```python
from build123d import *

# Parameters (mm, degrees)
BOSS_EXTRUDE1_DEPTH = 6.35
SKETCH3_R           = 3.302
SKETCH3_R_2         = 3.175
SKETCH3_R_3         = 7.14375
SKETCH3_R_4         = 1.905
CUT_EXTRUDE1_DEPTH  = 7.62
SKETCH5_R           = 2.667
SKETCH5_R_2         = 3.175
CUT_EXTRUDE2_DEPTH  = 7.62


with BuildPart() as part:
    # Sketch1 → Boss-Extrude1 (new body)
    with BuildSketch(Plane(origin=(0, 0, 0), x_dir=(1, 0, 0), z_dir=(0, 1, 0))):
        Polygon((0, 0), (495.3, 0), (495.3, -48.8188), (647.7, -48.8188), (647.7, 154.3812), (-152.4, 154.3812), (-152.4, -48.8188), (0, -48.8188), align=None)
    extrude(amount=BOSS_EXTRUDE1_DEPTH)

    # Sketch3 → Cut-Extrude1 (cut)
    with BuildSketch(Plane(origin=(0, 6.35, 0), x_dir=(1, 0, 0), z_dir=(0, 1, 0))):
        with Locations((-120.65, -15.7988)):
            Circle(SKETCH3_R)
        with Locations((-80.0608, 14.6304)):
            Circle(SKETCH3_R_2)
        with Locations((-123.825, 136.41832)):
            Circle(SKETCH3_R)
        with Locations((-80.0608, 147.9804)):
            Circle(SKETCH3_R_2)
        with Locations((21.463, 147.9804)):
            Circle(SKETCH3_R_2)
        with Locations((55.626, 73.1012)):
            Circle(SKETCH3_R_3)
        with Locations((619.125, 136.41832)):
            Circle(SKETCH3_R_2)
        with Locations((615.95, -15.7988)):
            Circle(SKETCH3_R_2)
        with Locations((580.009, 137.4648)):
            Circle(SKETCH3_R_4)
        with Locations((532.257, 94.4118)):
            Circle(SKETCH3_R_4)
        with Locations((580.009, 94.4118)):
            Circle(SKETCH3_R_4)
        with Locations((532.257, 136.41832)):
            Circle(SKETCH3_R_4)
        with Locations((439.674, 73.1012)):
            Circle(SKETCH3_R_3)
    extrude(amount=-CUT_EXTRUDE1_DEPTH, mode=Mode.SUBTRACT)

    # Sketch5 → Cut-Extrude2 (cut)
    with BuildSketch(Plane(origin=(0, 6.35, 0), x_dir=(1, 0, 0), z_dir=(0, 1, 0))):
        with Locations((120.65, 145.7452)):
            Circle(SKETCH5_R)
        with Locations((120.65, 41.3512)):
            Circle(SKETCH5_R)
        with Locations((419.1, 101.0412)):
            Circle(SKETCH5_R_2)
        with Locations((425.45, 22.3012)):
            Circle(SKETCH5_R_2)
        with Locations((361.95, 128.9812)):
            Circle(SKETCH5_R_2)
        with Locations((361.95, 22.3012)):
            Circle(SKETCH5_R_2)
        with Locations((302.9204, 145.7452)):
            Circle(SKETCH5_R)
        with Locations((302.9204, 41.3512)):
            Circle(SKETCH5_R)
        with Locations((133.35, 22.3012)):
            Circle(SKETCH5_R_2)
        with Locations((69.85, 22.3012)):
            Circle(SKETCH5_R_2)
    extrude(amount=-CUT_EXTRUDE2_DEPTH, mode=Mode.SUBTRACT)


solid = part.part
```
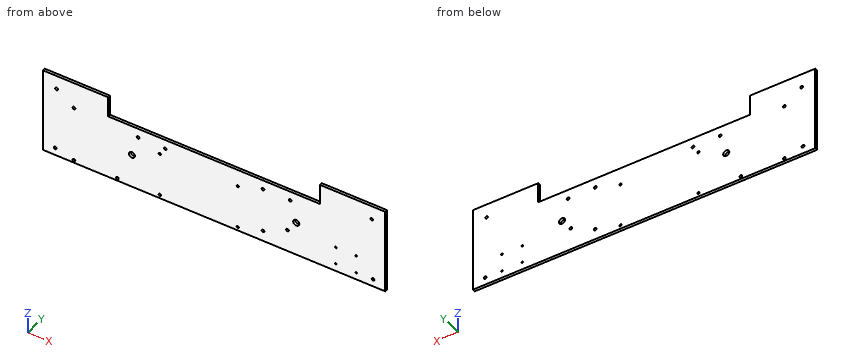
Check sheet for the modelled part. Datum: model origin and axes. Units: mm. Give positions to 0.01 mm unless a question says otherwise; leave off trailing zeros. Order: outer loops, then holes, each group sorted by start corner. A loop starts at its lowest first (then second) coordinate and runs counter-clockwise, first axis right, second up. Notation, with made-up numbers: M 57,65.25 L 100,65.25 A17 cw 100,84.25 Z; hole C 70.5,69.25 d4. An arc over 180 degrees is marked long. Answer in a Markdown table with one row per item. Add a question column.
Q1. Thickness scan on L1, parallel to Z at x = 120.65, y = 3.75; L2, parallel to X at y = 1.5, z = -94; L3, parallel to X at y = 1.25, z = 30. Record the ranges inside material, lowest first.
Q2. Gauge pin test, flat end, axial feed: pin 1 Ø5.5 at (x, z) = (-120.65, 15.8) entering from -Y. Record the tip position at first contact, or that the pin passes through.
Q3. Sectioned sample at A-A, the plane y = 2.25. Count the separate pieces of the cut face and the enclosed holes in it, and give its area (3 significant figures).
Q4. Sectioned sample at B-B, the plane x = 475. Record the boundary of the cut face in (y, z).
Verdict:
| question | item | result |
|---|---|---|
| 1 | L1 | -154.38 to -148.41, -143.08 to -44.02, -38.68 to 0 |
| 1 | L2 | -152.4 to 530.4, 534.12 to 578.15, 581.87 to 647.7 |
| 1 | L3 | -152.4 to 0, 495.3 to 647.7 |
| 2 | pin 1 | through |
| 3 | separate pieces | 1 |
| 3 | enclosed holes | 23 |
| 3 | area | 138,000 mm² |
| 4 | outline | M 0,-154.38 L 6.35,-154.38 L 6.35,0 L 0,0 Z |
